Build history of the part. All positions in model axes, mm. A direction names the side the tool comes from. Round coordinates to 2 decimals unless told otherwise and drop trailing zeros. Order: outer loops, then holes, each group sorted by start corner. A loop starts at its lowest first (then second) coordinate and runs counter-clockwise, first axis right, second up. Notation, with made-up numbers: M 53,30 L 71,30 A5 cw 71,35 Z; hole C -18,-5.5 d1. An arc over 180 degrees is marked long. One line per item, written item: value. Start each with the question number.
Item 1: Tool access for faces 1 (the flat face through (18, -17, 9.5)), 2 (the cylindrical face through (53.54, 29.08, 1.97)), 3 (the flat face through (18, -16, 1)), 4 (the flat face through (17, -59, 0)): list every direction of +Z, -Z, +X, -X, +Y, -Y with a clear straight run to the whole face (end or side of a thin tool).
Item 2: Band-saw the part on D-D, the plane x = 35.5. Write the cut outline in (y, z).
Item 3: Two-plate mould, pull along X, no slides. Class faces 5 (the flat face through (62.2, -18, 5)), 6 (the flat face through (47.7, 23.6, 4)), 7 (the flat face through (17, -72.796, 5)): +X half, -X half, draft (parallel to the pull), parting line (faces both ways), or undercut.
Item 4: Probe L1, parallel to Y at x = -15.15, z = 2.7; L2, parallel to Y at x = -15.15, z = 7.25; L3, parallel to X at y = 22, z = 2.75. List the from-to ranges inside material, lowest first.
Item 5: Pin check, flat tips, straight feed: pin 1 (4.5 mm diameter, centred on x = -15.15, y = 25.7, fed in from -Z); pin 2 (6 mm diameter, centred on x = 49.85, y = -59.3, fed in from -Z); pin 3 (5 mm diameter, centred on x = -6, y = -2.5, fed in from -Z). Stop position of each tip, or through.
Item 6: Band-saw the part on B-B, the plane y = -12.5. Write the cut outline in (x, z), then the cut area to 3 significant figures.
Item 7: Band-saw the part on A-A, the plane x = 49.85. Write the cut outline in (y, z).
Item 8: Band-saw the part on C-C, the plane x = 21. Write the cut outline in (y, z).
```python
from build123d import *

# Parameters (mm, degrees)
SKETCH_1_W          = 89.7
SKETCH_1_H          = 112
EXTRUDE_1_DEPTH     = 10.5
CUT_EXTRUDE_1_DEPTH = 1
CUT_EXTRUDE_2_DEPTH = 1
SKETCH_4_R          = 5
CUT_EXTRUDE_3_DEPTH = 4
SKETCH_15_R         = 2.5
CUT_EXTRUDE_4_DEPTH = 10


with BuildPart() as part:
    # 草图1 → 凸台-拉伸1 (new body)
    with BuildSketch(Plane.XY):
        with Locations((17.35, -16.795754715)):
            Rectangle(SKETCH_1_W, SKETCH_1_H)
    extrude(amount=EXTRUDE_1_DEPTH)

    # 草图2 → 切除-拉伸1 (cut)
    with BuildSketch(Plane.XY.offset(10.5)):
        Polygon((17.35, -1.595754715), (32.35, -1.595754715), (32.35, -31.995754715), (2.35, -31.995754715), (2.35, -1.595754715), align=None)
    extrude(amount=-CUT_EXTRUDE_1_DEPTH, mode=Mode.SUBTRACT)

    # 草图3 → 切除-拉伸2 (cut)
    with BuildSketch(Plane(origin=(0, 0, 0), x_dir=(-1, 0, 0), z_dir=(0, 0, -1))):
        Polygon((-62.2, -16.795754715), (-62.2, -44.795754715), (27.5, -44.795754715), (27.5, 11.204245285), (-62.2, 11.204245285), align=None)
    extrude(amount=-CUT_EXTRUDE_2_DEPTH, mode=Mode.SUBTRACT)

    # 草图4 → 切除-拉伸3 (cut)
    with BuildSketch(Plane(origin=(0, 0, 0), x_dir=(-1, 0, 0), z_dir=(0, 0, -1))):
        with Locations((-49.85, 25.704245285)):
            Circle(SKETCH_4_R)
        with Locations(Location((15.15, 25.704245285, 0), (0, 0, 180))):
            Circle(SKETCH_4_R)
        with Locations((15.15, -59.295754715)):
            Circle(SKETCH_4_R)
        with Locations(Location((-49.85, -59.295754715, 0), (0, 0, 180))):
            Circle(SKETCH_4_R)
    extrude(amount=-CUT_EXTRUDE_3_DEPTH, mode=Mode.SUBTRACT)

    # 草图15 → 切除-拉伸4 (cut)
    with BuildSketch(Plane(origin=(0, 0, 4), x_dir=(-1, 0, 0), z_dir=(0, 0, -1))):
        with Locations((-49.85, 25.704245285)):
            Circle(SKETCH_15_R)
        with Locations((15.15, 25.704245285)):
            Circle(SKETCH_15_R)
        with Locations((-49.85, -59.295754715)):
            Circle(SKETCH_15_R)
        with Locations((15.15, -59.295754715)):
            Circle(SKETCH_15_R)
    extrude(amount=-CUT_EXTRUDE_4_DEPTH, mode=Mode.SUBTRACT)


solid = part.part
```
Output:
1. face 1: +Z
1. face 2: -Z
1. face 3: -Z, +X, -X
1. face 4: -Z, +X, -X, +Y, -Y
2. outline: M -72.8,0 L -44.8,0 L -44.8,1 L 11.2,1 L 11.2,0 L 39.2,0 L 39.2,10.5 L -72.8,10.5 Z
3. face 5: +X half
3. face 6: undercut
3. face 7: draft
4. L1: y = -72.8 to -64.3, -54.3 to 20.7, 30.7 to 39.2
4. L2: y = -72.8 to -61.8, -56.8 to 23.2, 28.2 to 39.2
4. L3: x = -27.5 to -18.51, -11.79 to 46.49, 53.21 to 62.2
5. pin 1: passes through
5. pin 2: stops at z = 4
5. pin 3: stops at z = 1
6. outline: M -27.5,1 L 62.2,1 L 62.2,10.5 L 32.35,10.5 L 32.35,9.5 L 2.35,9.5 L 2.35,10.5 L -27.5,10.5 Z
6. area: 822 mm²
7. outline: M -72.8,0 L -64.3,0 L -64.3,4 L -61.8,4 L -61.8,10.5 L -72.8,10.5 Z; M -56.8,4 L -54.3,4 L -54.3,0 L -44.8,0 L -44.8,1 L 11.2,1 L 11.2,0 L 20.7,0 L 20.7,4 L 23.2,4 L 23.2,10.5 L -56.8,10.5 Z; M 28.2,4 L 30.7,4 L 30.7,0 L 39.2,0 L 39.2,10.5 L 28.2,10.5 Z
8. outline: M -72.8,0 L -44.8,0 L -44.8,1 L 11.2,1 L 11.2,0 L 39.2,0 L 39.2,10.5 L -1.6,10.5 L -1.6,9.5 L -32,9.5 L -32,10.5 L -72.8,10.5 Z
